```python
from build123d import *

# Parameters (mm, degrees)
SKETCH_1_R      = 3.3455
EXTRUDE_1_DEPTH = 6.8
CHAMFER_1_SIZE  = 0.6905


with BuildPart() as part:
    # Эскиз1 → Бобышка-Вытянуть1 (new body)
    with BuildSketch(Plane.XY):
        Polygon((-3.75277675, 6.5), (-7.505553499, 0), (-3.75277675, -6.5), (3.75277675, -6.5), (7.505553499, 0), (3.75277675, 6.5), align=None)
        Circle(SKETCH_1_R, mode=Mode.SUBTRACT)
    extrude(amount=EXTRUDE_1_DEPTH)

    # Фаска1
    chamfer_1_edges = [part.edges().sort_by_distance(p)[0] for p in [
        (-3.3455, 0, 0),
        (-3.3455, 0, 6.8),
    ]]
    chamfer(chamfer_1_edges, length=CHAMFER_1_SIZE)


solid = part.part
```
Model file for the job. Use its own axes, mm. Coordinates: 2 decimals unless noted, no trailing zeros. Order: outer loops, then holes, each group sorted by start corner. A loop starts at its lowest first (then second) coordinate and runs counter-clockwise, first axis right, second up. Notation, with made-up numbers: (-18.5, 67.5) -> (2.5, 67.5) arc R26 cw to (2.5, 85.5) -> close; hole circle Ø11 at (-38.75, 77). An arc over 180 degrees is marked (long way). Return JSON: item names as keys, results as strings.
Item 1: Slice it at C-C (y = 4.25). Write the cut outline in (x, z), then the cut area to 3 significant figures.
Model answer:
{"outline": "(-5.05, 0) -> (5.05, 0) -> (5.05, 6.8) -> (-5.05, 6.8) -> close", "area": "68.7 mm²"}
Item 2: Slice it at D-D (x = -6.5). Write the cut outline in (y, z), then the cut area to 3 significant figures.
Model answer:
{"outline": "(-1.74, 0) -> (1.74, 0) -> (1.74, 6.8) -> (-1.74, 6.8) -> close", "area": "23.7 mm²"}
Item 3: Wall check: line 1 along Y through (x, z) = (0, 4.9); line 2 along X through (y, z) = (-0.75, 4.25); line 3 along X through (y, z) = (3, 5.25). Give the ranges that are in metal, low to high. Write a range as from..to.
Model answer:
{"line 1": "y = -6.5..-3.35, 3.35..6.5", "line 2": "x = -7.07..-3.26, 3.26..7.07", "line 3": "x = -5.77..-1.48, 1.48..5.77"}
Item 4: Slice it at A-A (x = 0). Write the cut outline in (y, z).
Model answer:
{"outline": "(-6.5, 0) -> (-4.04, 0) -> (-3.35, 0.69) -> (-3.35, 6.11) -> (-4.04, 6.8) -> (-6.5, 6.8) -> close; (3.35, 0.69) -> (4.04, 0) -> (6.5, 0) -> (6.5, 6.8) -> (4.04, 6.8) -> (3.35, 6.11) -> close"}
Item 5: Pin check, flat tips, straight feed: P1, Ø1, axis at y = 3, z = 4, coming from the -X side; P2, Ø2, axis at x = -2.5, y = 0.5, coming from the -Z side. Stop position of each tip, or through.
Model answer:
{"P1": "stops at x = -6.06", "P2": "stops at z = 0.49"}
Item 6: Slice it at B-B (z = 2). Write the cut outline in (x, y), then the cut area to 3 significant figures.
Model answer:
{"outline": "(-7.51, 0) -> (-3.75, -6.5) -> (3.75, -6.5) -> (7.51, 0) -> (3.75, 6.5) -> (-3.75, 6.5) -> close; hole circle Ø6.69 at (0, 0)", "area": "111 mm²"}
Item 7: Mould opens along Y. For faces 1 (the face through (3, 3, 6.8)), 2 (the face through (-5.66, -3.2, 3.35)), 3 (the face through (-0.725, -3.266, 3.362)), 4 (the face through (-5.6, 3.3, 3.4)) say: pulls with the +Y half, pulls with the -Y half, needs draft (parallel to the pull), parting line crosses it, or undercut.
Model answer:
{"face 1": "needs draft", "face 2": "pulls with the -Y half", "face 3": "undercut", "face 4": "pulls with the +Y half"}
